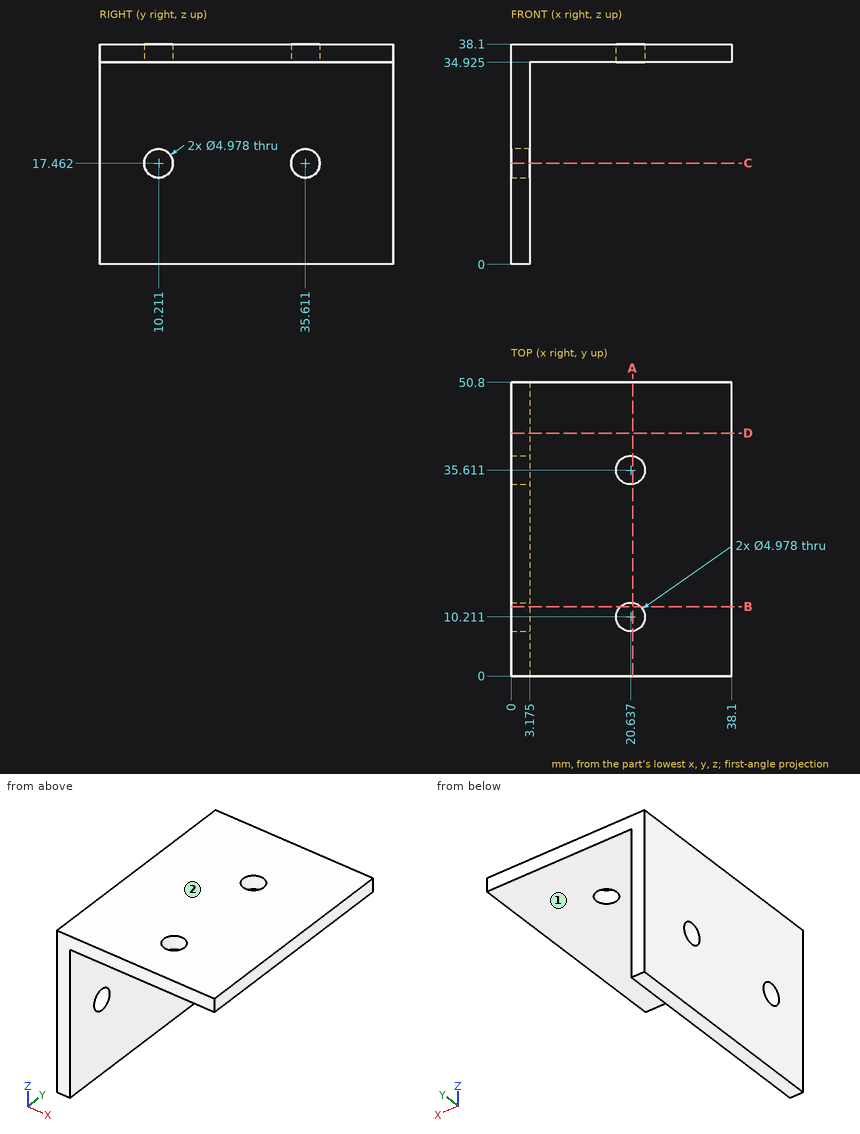
Input: dimensioned drawing with shaded views. Units: mm. Origin: part minimum x, y, z. A direction names the side the tool comes from. Give positions to 0.01 mm unless a question says otherwise; leave off trailing zeros. Write each loop counter-clockwise with the first axis right and the second up, starting at its lowest first coordinate (ties: lowest second). Pieces come first, ordered by that corner, then holes.
Q1. First-contact query: P1, Ø12, axis at x = 13.5, y = 34, coming from the -Z side (1 decimal); P2, Ø8, axis at x = 28.5, z = 34, coming from the -Y side; P3, Ø4.5, axis at x = 20.64, y = 35.61, coming from the -Z side; P4, Ø3, axis at y = 10, z = 19, coming from the +X side (1 decimal). Flat tips, straight axial feed; report the tip coordinate or a pass-through.
Q2. Section D-D, the plane y = 42. Output: boundary loops of the cut face in (x, z) (1 decimal).
Q3. Section A-A, the plane x = 21. Output: boundary loops of the cut face in (y, z) (1 decimal), plus the area to 3 significant figures.
Q4. Section B-B, the plane y = 12. Output: boundary loops of the cut face in (x, z) (1 decimal).
Q5. Material intervals for probe 1 along Z at (x, y) = (15.5, 25.5) (1 decimal); probe 2 along X at (y, z) = (7.5, 11.5) (1 decimal), sorted ascending.
Q6. Section C-C, the plane z = 17.5. Output: boundary loops of the cut face in (x, y) (1 decimal), plus the area to 3 significant figures.
Q7. Set-up query: the marked faces 1 and 2. Return all of +Z, -Z, +X, -X, +Y, -Y with unobstructed straight access to the full face (end or side cutting, diameter ignored); none if empty.
Filled in:
1. P1: stops at z = 34.9
1. P2: stops at y = 0
1. P3: passes through
1. P4: stops at x = 3.2
2. outline: (0, 0) - (3.2, 0) - (3.2, 34.9) - (38.1, 34.9) - (38.1, 38.1) - (0, 38.1) - close
3. outline: (0, 34.9) - (7.7, 34.9) - (7.7, 38.1) - (0, 38.1) - close; (12.7, 34.9) - (33.1, 34.9) - (33.1, 38.1) - (12.7, 38.1) - close; (38.1, 34.9) - (50.8, 34.9) - (50.8, 38.1) - (38.1, 38.1) - close
3. area: 130 mm2
4. outline: (0, 0) - (3.2, 0) - (3.2, 15.7) - (0, 15.7) - close; (0, 19.2) - (3.2, 19.2) - (3.2, 34.9) - (18.9, 34.9) - (18.9, 38.1) - (0, 38.1) - close; (22.4, 34.9) - (38.1, 34.9) - (38.1, 38.1) - (22.4, 38.1) - close
5. probe 1: z = 34.9 to 38.1
5. probe 2: x = 0 to 3.2
6. outline: (0, 0) - (3.2, 0) - (3.2, 7.7) - (0, 7.7) - close; (0, 12.7) - (3.2, 12.7) - (3.2, 33.1) - (0, 33.1) - close; (0, 38.1) - (3.2, 38.1) - (3.2, 50.8) - (0, 50.8) - close
6. area: 130 mm2
7. face 1: -Z, +X, +Y, -Y
7. face 2: +Z, +X, -X, +Y, -Y
